```python
from build123d import *

# Parameters (mm, degrees)
CROQUIS1_W              = 70
CROQUIS1_H              = 110
SALIENTE_EXTRUIR1_DEPTH = 5
CROQUIS2_W              = 15
CROQUIS2_H              = 30
CORTAR_EXTRUIR1_DEPTH   = 99.417594391


with BuildPart() as part:
    # Croquis1 → Saliente-Extruir1 (new body)
    with BuildSketch(Plane(origin=(0, 0, 0), x_dir=(1, 0, 0), z_dir=(0, 1, 0))):
        with Locations((19.079422383, -27.075812274)):
            Rectangle(CROQUIS1_W, CROQUIS1_H)
    extrude(amount=SALIENTE_EXTRUIR1_DEPTH)

    # Croquis2 → Cortar-Extruir1 (cut, through all)
    with BuildSketch(Plane(origin=(0, 5, 0), x_dir=(1, 0, 0), z_dir=(0, 1, 0))):
        with Locations((-8.420577617, -40.075812274)):
            Rectangle(CROQUIS2_W, CROQUIS2_H)
    extrude(amount=-CORTAR_EXTRUIR1_DEPTH, mode=Mode.SUBTRACT)


solid = part.part
```
Can you work these out from the model? Positions are in its coordinate system, mm. A direction names the side the tool comes from. Round coordinates to 2 decimals unless told otherwise and drop trailing zeros. Loops run counter-clockwise (first coordinate to the right, second up) from the corner with the lowest first, then second, coordinate; pieces in that order, holes last. Notation, with made-up numbers: M 67,37.25 L 122,37.25 A17 ccw 122,49.25 Z; hole C 65,-3.5 d7. An arc over 180 degrees is marked long. Answer in a Markdown table with one row per item.
1. If we section it at A-A, the plane x = -3.5: Please give me the cut outline in (y, z), plus the area to 3 significant figures.
Established:
| item | result |
|---|---|
| outline | M 0,-27.92 L 5,-27.92 L 5,25.08 L 0,25.08 Z; M 0,55.08 L 5,55.08 L 5,82.08 L 0,82.08 Z |
| area | 400 mm² |
2. I'm going to push a flat-ended pin straight in: pin 1 Ø1.5 at (y, z) = (1.5, 34) entering from -X. Where does the tip first touch, or does it pass through?
Established:
| item | result |
|---|---|
| pin 1 | x = -0.92 |
3. Please list where these lines run through material, in increasing order: line 1 (Z direction, x = -4, y = 2.7); line 2 (X direction, y = 0.95, z = 49.5). Write a range as from..to.
Established:
| item | result |
|---|---|
| line 1 | -27.92..25.08, 55.08..82.08 |
| line 2 | -0.92..54.08 |
4. Thinking about a two-plate mould opening in Z: for faces 1 (the face through (19, 2, -27.924)), 2 (the face through (19, 2, 82.076)), 3 (the face through (-0.921, 3, 40)), which applies, pulls with the +Z half, pulls with the -Z half, needs draft (parallel to the pull), parting line crosses it, or undercut?
Established:
| item | result |
|---|---|
| face 1 | pulls with the -Z half |
| face 2 | pulls with the +Z half |
| face 3 | undercut |
5. If we section it at B-B, the plane y = 3.45: Please give me the cut outline in (x, z), plus the area to 3 significant figures.
Established:
| item | result |
|---|---|
| outline | M -15.92,-27.92 L 54.08,-27.92 L 54.08,82.08 L -15.92,82.08 L -15.92,55.08 L -0.92,55.08 L -0.92,25.08 L -15.92,25.08 Z |
| area | 7,250 mm² |
6. On a 3-axis mill with a long thin cutter (end or side, diameter ignored), from which of +Z, -Z, +X, -X, +Y, -Y can I reach the whole of each face in a straight line? I mean faces 4 (the face through (-9, 3, 55.076)), 5 (the face through (19, 0, 26)). Say none if no direction works.
Established:
| item | result |
|---|---|
| face 4 | -X, +Y, -Y |
| face 5 | +Z, -Z, +X, -X, -Y |
